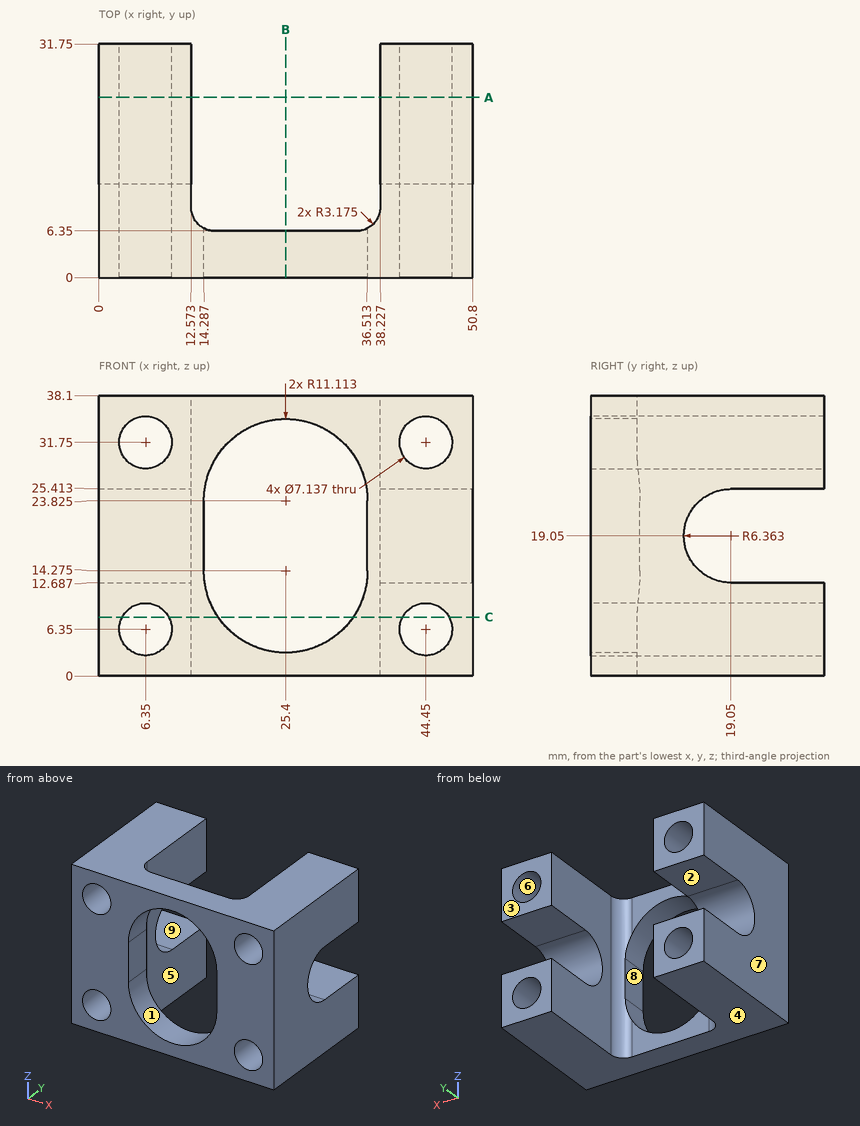
Source: three-view drawing plus pictorial views. Frame: mm from the lowest corner of the part. A direction names the side the tool comes from. Coordinates: 2 decimals unless noted, no trailing zeros. Loops run counter-clockwise (first coordinate to the right, second up) from the corner with the lowest first, then second, coordinate; pieces in that order, holes last. Notation, with made-up numbers: (-37.5, 26) - (11.5, 26) arc R25 cw to (11.5, 40) - close; hole circle Ø10 at (-29, 29). An arc over 180 degrees is marked (long way). One line per item, written item: value. Start each with the question number.
1. Mould query, pull axis X, two halves, no side actions, for the marked faces 6, 7, 8 and 9. Classes: pulls with the +X half, pulls with the -X half, needs draft (parallel to the pull), parting line crosses it, or undercut.
2. Section B-B (x = 25.4). Return the cut outline in (y, z).
3. Section C-C (z = 8). State how many separate pieces and enclosed holes the cut face has.
4. Set-up query: the marked faces 1, 2, 3, 4 and 5. Return all of +Z, -Z, +X, -X, +Y, -Y with unobstructed straight access to the full face (end or side cutting, diameter ignored); none if empty.
5. Contact query for flat-ended pins moving along their axis: P1, Ø7, axis at x = 29, z = 2.5, coming from the +Y side; P2, Ø3, axis at x = 43.5, z = 31, coming from the -Y side. Output: stop coordinate, or through.
6. Ray query, L1, parallel to X at y = 25, z = 31.75; L2, parallel to X at y = 2.5, z = 23; L3, parallel to X at y = 27.5, z = 36. Return the intervals inside material, ascending.
7. Section A-A (y = 24.5). Return the cut outline in (x, z), and give its area (3 significant figures).
Verdict:
1. face 6: undercut
1. face 7: pulls with the -X half
1. face 8: undercut
1. face 9: needs draft
2. outline: (0, 0) - (6.35, 0) - (6.35, 3.16) - (0, 3.16) - close; (0, 34.94) - (6.35, 34.94) - (6.35, 38.1) - (0, 38.1) - close
3. separate pieces: 4
3. enclosed holes: 0
4. face 1: +Y, -Y
4. face 2: +X, -X, +Y
4. face 3: +Z, -Z, +X, -X, +Y
4. face 4: -Z, +X, -X, +Y, -Y
4. face 5: +Z, -Z, +Y
5. P1: stops at y = 6.35
5. P2: passes through
6. L1: x = 0 to 2.78, 9.92 to 12.57, 38.23 to 40.88, 48.02 to 50.8
6. L2: x = 0 to 14.29, 36.51 to 50.8
6. L3: x = 0 to 12.57, 38.23 to 50.8
7. outline: (0, 0) - (12.57, 0) - (12.57, 12.69) - (0, 12.69) - close; (0, 25.41) - (12.57, 25.41) - (12.57, 38.1) - (0, 38.1) - close; (38.23, 0) - (50.8, 0) - (50.8, 12.69) - (38.23, 12.69) - close; (38.23, 25.41) - (50.8, 25.41) - (50.8, 38.1) - (38.23, 38.1) - close; hole circle Ø7.14 at (6.35, 6.35); hole circle Ø7.14 at (6.35, 31.75); hole circle Ø7.14 at (44.45, 6.35); hole circle Ø7.14 at (44.45, 31.75)
7. area: 478 mm2
